```python
from build123d import *

# Parameters (mm, degrees)
CROQUIS1_R              = 16
SALIENTE_EXTRUIR1_DEPTH = 13
VACIADO1_T              = -2
CROQUIS2_W              = 7.778512226
CROQUIS2_H              = 19.595917942
CROQUIS2_W_2            = 8.965433382
CORTAR_EXTRUIR1_DEPTH   = 10
SALIENTE_EXTRUIR2_REACH = 28.096
CROQUIS3_W              = 2.5
CROQUIS3_H              = 19.595917942
CROQUIS4_R              = 1.1
CORTAR_EXTRUIR2_DEPTH   = 36.174564674
CROQUIS5_R              = 1.1
CORTAR_EXTRUIR3_DEPTH   = 47.786750261
C_PULA1_FACE_RADIUS     = 16
C_PULA1_HEIGHT          = 3
CROQUIS7_R              = 7.9
CORTAR_EXTRUIR4_DEPTH   = 10


with BuildPart() as part:
    # Croquis1 → Saliente-Extruir1 (new body)
    with BuildSketch(Plane(origin=(0, 0, 0), x_dir=(1, 0, 0), z_dir=(0, 1, 0))):
        with Locations(Location((0, 0, 0), (0, 0, 90))):
            Circle(CROQUIS1_R)
    extrude(amount=SALIENTE_EXTRUIR1_DEPTH)

    # Vaciado1
    vaciado1_openings = [part.faces().sort_by_distance(p)[0] for p in [
        (0, 0, 0),
    ]]
    offset(amount=VACIADO1_T, openings=vaciado1_openings, kind=Kind.INTERSECTION)

    # Croquis2 → Cortar-Extruir1 (cut)
    with BuildSketch(Plane.XZ):
        with Locations((13.889256113, 0)):
            Rectangle(CROQUIS2_W, CROQUIS2_H)
        with Locations((-14.482716691, 0)):
            Rectangle(CROQUIS2_W_2, CROQUIS2_H)
    extrude(amount=-CORTAR_EXTRUIR1_DEPTH, mode=Mode.SUBTRACT)

    # Croquis3 → Saliente-Extruir2 (add, up to next)
    with BuildSketch(Plane.XZ, mode=Mode.PRIVATE) as saliente_extruir2_sk1:
        with Locations((-11.25, 0)):
            Rectangle(CROQUIS3_W, CROQUIS3_H)
    saliente_extruir2_tool1 = extrude(saliente_extruir2_sk1.sketch, amount=-SALIENTE_EXTRUIR2_REACH, mode=Mode.PRIVATE) - part.part
    # Croquis3 → Saliente-Extruir2 (add, up to next)
    with BuildSketch(Plane.XZ, mode=Mode.PRIVATE) as saliente_extruir2_sk2:
        with Locations((11.25, 0)):
            Rectangle(CROQUIS3_W, CROQUIS3_H)
    saliente_extruir2_tool2 = extrude(saliente_extruir2_sk2.sketch, amount=-SALIENTE_EXTRUIR2_REACH, mode=Mode.PRIVATE) - part.part
    add(saliente_extruir2_tool1.solids().sort_by_distance((-11.25, 0, 0))[0])
    add(saliente_extruir2_tool2.solids().sort_by_distance((11.25, 0, 0))[0])

    # Croquis4 → Cortar-Extruir2 (cut, through all)
    with BuildSketch(Plane.ZY.offset(12.5)):
        with Locations((0, 7.9)):
            Circle(CROQUIS4_R)
    extrude(amount=-CORTAR_EXTRUIR2_DEPTH, mode=Mode.SUBTRACT)

    # Croquis5 → Cortar-Extruir3 (cut, through all)
    with BuildSketch(Plane.XY.offset(26)):
        with Locations((0, 4)):
            Circle(CROQUIS5_R)
    extrude(amount=-CORTAR_EXTRUIR3_DEPTH, mode=Mode.SUBTRACT)

    # Cúpula1: a dome of height H over a round flat face of radius A is a cap of a sphere of radius (A * A + H * H) / (2 * H)
    c_pula1_r = (C_PULA1_FACE_RADIUS * C_PULA1_FACE_RADIUS + C_PULA1_HEIGHT * C_PULA1_HEIGHT) / (2 * C_PULA1_HEIGHT)
    c_pula1_base = Plane((0, 13, 0), z_dir=(0, 1, 0))
    with Locations(c_pula1_base.offset(C_PULA1_HEIGHT - c_pula1_r)):
        c_pula1_ball = Sphere(c_pula1_r, mode=Mode.PRIVATE)
    add(split(c_pula1_ball, bisect_by=c_pula1_base, keep=Keep.TOP, mode=Mode.PRIVATE))

    # Croquis7 → Cortar-Extruir4 (cut)
    with BuildSketch(Plane.XZ.offset(-11)):
        with Locations(Location((0, 0, 0), (0, 0, 270))):
            Circle(CROQUIS7_R)
    extrude(amount=-CORTAR_EXTRUIR4_DEPTH, mode=Mode.SUBTRACT)


solid = part.part
```
Geometry check sheet. Reference: the model listing, model coordinates, mm. A direction names the side the tool comes from. Round coordinates to 2 decimals unless told otherwise and drop trailing zeros. Loops run counter-clockwise (first coordinate to the right, second up) from the corner with the lowest first, then second, coordinate; pieces in that order, holes last. Notation, with made-up numbers: (-33.5, -11) -> (4.5, -11) arc R15 ccw to (4.5, 10) -> close; hole circle Ø2 at (78, 22). An arc over 180 degrees is marked (long way). Use a Markdown table: item, result.
(1) Go/stop test with flat-tipped pins: P1, Ø4, axis at x = 7, z = 2.5, coming from the -Y side; P2, Ø2.5, axis at y = 7.9, z = 0, coming from the +X side; P3, Ø1.2, axis at x = -13.5, z = 3, coming from the -Y side. Record where each tip stops, or that it passes through.
Calculated:
| item | result |
|---|---|
| P1 | y = 11 |
| P2 | x = 12.5 |
| P3 | y = 10 |
(2) Sectioned sample at C-C (z = 0). Enter the section's corners in (x, y).
Calculated:
| item | result |
|---|---|
| outline | (-16, 10) -> (-14, 10) -> (-14, 11) -> (-12.5, 11) -> (-12.5, 9) -> (-10, 9) -> (-10, 11) -> (-7.9, 11) -> (-7.9, 15.29) arc R44.17 ccw to (-16, 13) -> close; (-12.5, 0) -> (-10, 0) -> (-10, 6.8) -> (-12.5, 6.8) -> close; (7.9, 11) -> (10, 11) -> (10, 9) -> (12.5, 9) -> (12.5, 11) -> (14, 11) -> (14, 10) -> (16, 10) -> (16, 13) arc R44.17 ccw to (7.9, 15.29) -> close; (10, 0) -> (12.5, 0) -> (12.5, 6.8) -> (10, 6.8) -> close |
(3) Scan lines: probe 1 along X at (y, z) = (5.5, -12); probe 2 along Z at (x, y) = (-3, 6); probe 3 along Z at (x, y) = (6, 7.75). Record each from-to range of solid material in increasing order.
Calculated:
| item | result |
|---|---|
| probe 1 | -10.58 to -7.21, 7.21 to 10.58 |
| probe 2 | -15.72 to -13.67, 13.67 to 15.72 |
| probe 3 | -14.83 to -12.65, 12.65 to 14.83 |
(4) Sectioned sample at A-A (x = 0). Enter the section's corners in (y, z), then the cut area to 3 significant figures.
Calculated:
| item | result |
|---|---|
| outline | (0, -16) -> (2.9, -16) -> (2.9, -14) -> (0, -14) -> close; (0, 14) -> (2.9, 14) -> (2.9, 16) -> (0, 16) -> close; (5.1, -16) -> (13, -16) arc R44.17 ccw to (15.29, -7.9) -> (11, -7.9) -> (11, -14) -> (5.1, -14) -> close; (5.1, 14) -> (11, 14) -> (11, 7.9) -> (15.29, 7.9) arc R44.17 ccw to (13, 16) -> (5.1, 16) -> close |
| area | 88.4 mm² |
(5) Sectioned sample at D-D (x = -4). Enter the section's corners in (y, z), then the cut area to 3 significant figures.
Calculated:
| item | result |
|---|---|
| outline | (0, -15.49) -> (13, -15.49) arc R43.99 ccw to (15.29, -6.81) -> (11, -6.81) -> (11, -13.42) -> (0, -13.42) -> close; (0, 13.42) -> (11, 13.42) -> (11, 6.81) -> (15.29, 6.81) arc R43.99 ccw to (13, 15.49) -> (0, 15.49) -> close |
| area | 103 mm² |
(6) Mould release check, pull along X, two halves, no side actions. Record for faces 1 (the cylindrical face through (-0.703, 7.853, 15.985)), 2 (the flat face through (10.2, 0, 0.1)), 3 (the cylindrical face through (0.59, 4.93, 14.99)): released by +X, released by -X, zero draft, split by the parting line, or undercut.
Calculated:
| item | result |
|---|---|
| face 1 | split by the parting line |
| face 2 | zero draft |
| face 3 | undercut |
(7) Sectioned sample at B-B (y = 7.9). Enter the section's corners in (x, z).
Calculated:
| item | result |
|---|---|
| outline | (-12.65, -9.8) arc R16 ccw to (12.65, -9.8) -> (12.5, -9.8) -> (12.5, -1.1) -> (10, -1.1) -> (10, -9.8) arc R14 cw to (-10, -9.8) -> (-10, -1.1) -> (-12.5, -1.1) -> (-12.5, -9.8) -> close; (-12.65, 9.8) -> (-12.5, 9.8) -> (-12.5, 1.1) -> (-10, 1.1) -> (-10, 9.8) arc R14 cw to (10, 9.8) -> (10, 1.1) -> (12.5, 1.1) -> (12.5, 9.8) -> (12.65, 9.8) arc R16 ccw to start |
(8) Set-up check for faces 4 (the flat face through (13, 11, 0)), 5 (the cylindrical face through (5.34, 13.11, 5.82)): record each of +Z, -Z, +X, -X, +Y, -Y from which the full face is reachable in a straight line by a thin tool's end or side.
Calculated:
| item | result |
|---|---|
| face 4 | -Y |
| face 5 | +Y, -Y |
